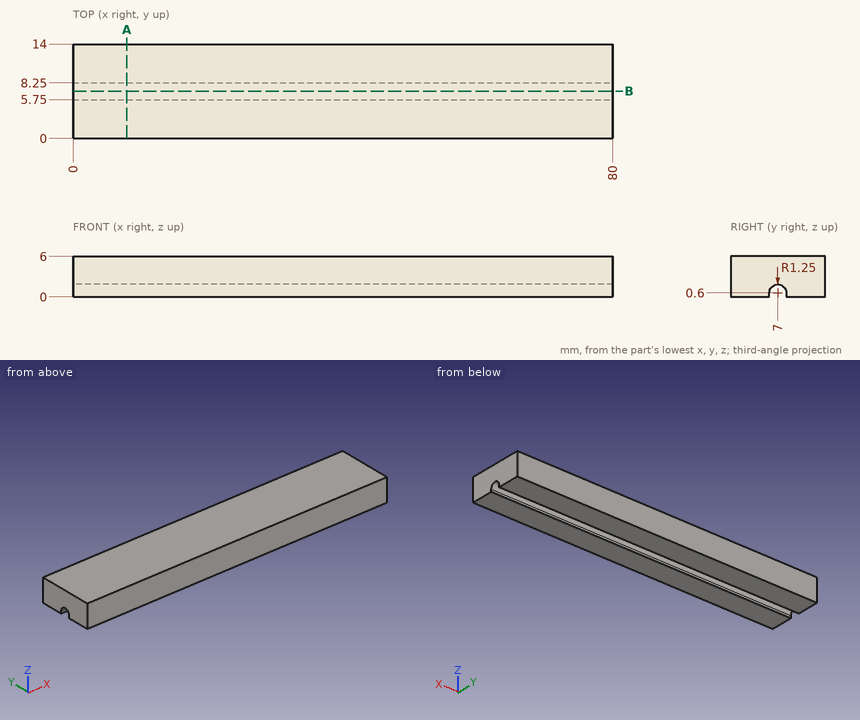
Here's the drawing with two shaded views (mm, measured from the low corner). I have some questions. Coordinates: 2 decimals unless noted, no trailing zeros. Order: outer loops, then holes, each group sorted by start corner. A loop starts at its lowest first (then second) coordinate and runs counter-clockwise, first axis right, second up. Notation, with made-up numbers: M 28,18 L 56,18 A12 cw 56,35 Z; hole C 19.25,-34 d1. An arc over 180 degrees is marked long. Write item = value, one per line.
(1) Suppose I cut it at B-B on y = 7. Please give me the cut outline in (x, z).
Results are:
outline = M 0,1.85 L 80,1.85 L 80,6 L 0,6 Z
(2) Suppose I cut it at A-A on x = 8. Please give me the cut outline in (y, z), plus the area to 3 significant figures.
Results are:
outline = M 0,0 L 5.75,0 L 5.75,0.6 A1.25 cw 8.25,0.6 L 8.25,0 L 14,0 L 14,6 L 0,6 Z
area = 80.0 mm2
(3) For pin 1 Ø2 at (y, z) = (11, 3.5) entering from -X, with a flat end and sliding along its axis, tell me the tip position at first contact or that it passes through.
Results are:
pin_1 = 0
(4) I need wall thicknesses on line 1 along Y through (x, z) = (52.5, 1.05); line 2 along Y through (x, z) = (34, 1.1); line 3 along Z through (x, y) = (48, 6). Which ranges of each line are inside material? Lowest first, please. Write a range as [from, to].
Results are:
line_1 = [0, 5.83], [8.17, 14]
line_2 = [0, 5.85], [8.15, 14]
line_3 = [1.35, 6]
